Work out the finished part from the listing and answer in its coordinate system (mm). A direction names the side the tool comes from. Round coordinates to 2 decimals unless told otherwise and drop trailing zeros. Order: outer loops, then holes, each group sorted by start corner. A loop starts at its lowest first (then second) coordinate and runs counter-clockwise, first axis right, second up. Notation, with made-up numbers: (26.25, 59.5) - (83.25, 59.5) arc R26 ccw to (83.25, 96.5) - close; hole circle Ø1 at (-13.5, 2). An arc over 180 degrees is marked (long way). One line per question, with ' | ' between items. Start each with the question number.
Solid Edge part; units mm, degrees
sketch "Sketch1" plane through (0, 0, 0) normal (0, 0, 1) x (1, 0, 0)
  line L0 (15.9526, 57.5957) -> (0, 57.5957)
  line L1 (0, 22.5957) -> (0, 57.5957)
  line L2 (0, 22.5957) -> (15.7947, 22.5957)
  arc A0 (15.9526, 57.5957) -> (15.7947, 22.5957) centre (37.0865, 40) cw
  circle A1 centre (37.0865, 40) radius 16.65
extrude "Protrusion1" add sketch "Sketch1" along normal blind 2
1) Section B-B on z = 0.9 is taken. Give the vertices of the cut face in (x, y), and give its area (3 significant figures).
2) Determine the mould class of faces 1 (the flat face through (0, 40, 1)), 2 (the cylindrical face through (46.04, 25.96, 0.99)), 3 (the flat face through (8, 22.596, 1)) for opening direction X: released by +X, released by -X, zero draft, split by the parting line, or undercut.
3) A flat-ended cylindrical pin translates along its axis: pin 1 (0.6 mm diameter, centred on x = 11.5, z = 0.5, fed in from +Y). Find the tip coordinate at first contact, or state that the pin passes through.
4) Straight lines are drawn through the part: line 1 (Y direction, x = 36.5, z = 0.35); line 2 (Y direction, x = 4.5, z = 0.25); line 3 (X direction, y = 50, z = 1.5). For each, find the intervals that lie inside material, in ascending order.
5) Section A-A on y = 40 is taken. Give the vertices of the cut face in (x, z).
6) Section C-C on x = 45.5 is taken. Give the vertices of the cut face in (y, z), and give its area (3 significant figures).
7) For faces 4 (the flat face through (25, 28, 0)), 5 (the flat face through (8, 57.596, 1)), determine the directions among +Z, -Z, +X, -X, +Y, -Y from which every point of the face is accessible in a straight line to the end or side of a thin tool.
8) Section D-D on y = 63.5 is taken. Give the vertices of the cut face in (x, z).
Recorded:
1) outline: (0, 22.6) - (15.79, 22.6) arc R27.5 ccw (long way) to (15.95, 57.6) - (0, 57.6) - close; hole circle Ø33.3 at (37.09, 40) | area: 1,910 mm²
2) face 1: released by -X | face 2: undercut | face 3: zero draft
3) pin 1: stops at y = 57.6
4) line 1: y = 12.51 to 23.36, 56.64 to 67.49 | line 2: y = 22.6 to 57.6 | line 3: x = 0 to 23.77, 50.4 to 62.7
5) outline: (0, 0) - (20.44, 0) - (20.44, 2) - (0, 2) - close; (53.74, 0) - (64.59, 0) - (64.59, 2) - (53.74, 2) - close
6) outline: (13.82, 0) - (25.63, 0) - (25.63, 2) - (13.82, 2) - close; (54.37, 0) - (66.18, 0) - (66.18, 2) - (54.37, 2) - close | area: 47.3 mm²
7) face 4: -Z, +X, -X, +Y, -Y | face 5: +Z, -Z, -X, +Y
8) outline: (22.8, 0) - (51.37, 0) - (51.37, 2) - (22.8, 2) - close
